```python
from build123d import *

# Parameters (mm, degrees)
SKETCH1_W           = 95.192719723
SKETCH1_H           = 77.236030742
BOSS_EXTRUDE1_DEPTH = 5
SKETCH2_W           = 20.458340989
SKETCH2_H           = 77.236030742
BOSS_EXTRUDE2_DEPTH = 2
SKETCH3_W           = 97.192719723
SKETCH3_H           = 20.458340989
BOSS_EXTRUDE3_DEPTH = 2
SKETCH4_W           = 97.192719723
SKETCH4_H           = 20.458340989
BOSS_EXTRUDE4_DEPTH = 2
LPATTERN1_COUNT     = 6
LPATTERN1_PITCH     = 19.038543945
CUT_EXTRUDE1_REACH  = 115.159
SKETCH7_W           = 11.458340989
SKETCH7_H           = 3.5


with BuildPart() as part:
    # Sketch1 → Boss-Extrude1 (new body)
    with BuildSketch(Plane.XY):
        with Locations((47.596359862, -38.618015371)):
            Rectangle(SKETCH1_W, SKETCH1_H)
    extrude(amount=BOSS_EXTRUDE1_DEPTH)

    # Sketch2 → Boss-Extrude2 (add)
    with BuildSketch(Plane.ZY):
        with Locations((10.229170494, -38.618015371)):
            Rectangle(SKETCH2_W, SKETCH2_H)
    boss_extrude2 = extrude(amount=BOSS_EXTRUDE2_DEPTH)

    # Sketch3 → Boss-Extrude3 (add)
    with BuildSketch(Plane(origin=(0, 0, 0), x_dir=(1, 0, 0), z_dir=(0, 1, 0))):
        with Locations((46.596359862, -10.229170494)):
            Rectangle(SKETCH3_W, SKETCH3_H)
    extrude(amount=BOSS_EXTRUDE3_DEPTH)

    # Sketch4 → Boss-Extrude4 (add)
    with BuildSketch(Plane.XZ.offset(77.236030742)):
        with Locations((46.596359862, 10.229170494)):
            Rectangle(SKETCH4_W, SKETCH4_H)
    extrude(amount=BOSS_EXTRUDE4_DEPTH)

    # LPattern1: Boss-Extrude2 ×6
    with Locations(*[(i * LPATTERN1_PITCH, 0, 0) for i in range(1, LPATTERN1_COUNT)]):
        add(boss_extrude2)

    # Cut-Extrude1: up to this face of the body (flat: up to its plane)
    cut_extrude1_end = Plane(part.part.faces().sort_by_distance((76.154175778, -38.618015371, 12.729170494))[0])
    # Sketch7 → Cut-Extrude1 (cut, up to the picked face)
    with BuildSketch(Plane.ZY.offset(-17.038543945), mode=Mode.PRIVATE) as cut_extrude1_sk1:
        with Locations((12.729170494, -1.75)):
            Rectangle(SKETCH7_W, SKETCH7_H)
    cut_extrude1_tool1 = split(extrude(cut_extrude1_sk1.sketch, amount=-CUT_EXTRUDE1_REACH, mode=Mode.PRIVATE), bisect_by=cut_extrude1_end, keep=Keep.BOTH, mode=Mode.PRIVATE)
    # Sketch7 → Cut-Extrude1 (cut, up to the picked face)
    with BuildSketch(Plane.ZY.offset(-17.038543945), mode=Mode.PRIVATE) as cut_extrude1_sk2:
        with Locations((12.729170494, -75.486030742)):
            Rectangle(SKETCH7_W, SKETCH7_H)
    cut_extrude1_tool2 = split(extrude(cut_extrude1_sk2.sketch, amount=-CUT_EXTRUDE1_REACH, mode=Mode.PRIVATE), bisect_by=cut_extrude1_end, keep=Keep.BOTH, mode=Mode.PRIVATE)
    add(cut_extrude1_tool1.solids().sort_by(Axis((17.038544, -1.75, 12.72917), (1, 0, 0)))[0], mode=Mode.SUBTRACT)
    add(cut_extrude1_tool2.solids().sort_by(Axis((17.038544, -75.486031, 12.72917), (1, 0, 0)))[0], mode=Mode.SUBTRACT)


solid = part.part
```
Geometry check sheet. Reference: the model listing, model coordinates, mm. A direction names the side the tool comes from. Round coordinates to 2 decimals unless told otherwise and drop trailing zeros. Order: outer loops, then holes, each group sorted by start corner. A loop starts at its lowest first (then second) coordinate and runs counter-clockwise, first axis right, second up. Notation, with made-up numbers: (21, -5.5) - (70, -5.5) arc R24 ccw to (70, 6.5) - close; hole circle Ø9 at (-11.75, 27.25). An arc over 180 degrees is marked (long way). Use a Markdown table: item, result. Add a question column.
1) Thickness scan on line 1 along X through (y, z) = (-73, 16.75); line 2 along Y through (x, z) = (56.5, 17.75); line 3 along Y through (x, z) = (87, 10.5). Record the ranges inside material, lowest first.
2) Mould release check, pull along Z, two halves, no side actions. Record for faces 1 (the flat face through (46, 2, 10)), 2 (the flat face through (18, -76, 18.458)), 3 (the flat face through (8, -38, 5)): released by +Z, released by -Z, zero draft, split by the parting line, or undercut.
3) Set-up check for faces 4 (the flat face through (75, -3.5, 13)), 5 (the flat face through (19.039, -38, 13)): record each of +Z, -Z, +X, -X, +Y, -Y from which the full face is reachable in a straight line by a thin tool's end or side.
4) Section check C-C (x = 61.5). Record the cut outline in (y, z), then the cut area to 3 significant figures.
5) Section check B-B (y = -54). Record the cut outline in (x, z), then the cut area to 3 significant figures.
6) Section check A-A (z = 15.5). Record the cut outline in (x, y).
7) Gauge pin test, flat ends, axial feed: P1, Ø6, axis at x = 13.5, y = -68.5, coming from the +Z side; P2, Ø18.5, axis at x = 46.5, y = -48.5, coming from the +Z side. Record the tip position at first contact, or that the pin passes through.
Established:
| question | item | result |
|---|---|---|
| 1 | line 1 | -2 to 0, 17.04 to 19.04, 36.08 to 38.08, 55.12 to 57.12, 74.15 to 76.15, 93.19 to 95.19 |
| 1 | line 2 | -79.24 to -77.24, -73.74 to -3.5, 0 to 2 |
| 1 | line 3 | -79.24 to -77.24, 0 to 2 |
| 2 | face 1 | zero draft |
| 2 | face 2 | undercut |
| 2 | face 3 | released by +Z |
| 3 | face 4 | none |
| 3 | face 5 | +Z |
| 4 | outline | (-79.24, 0) - (2, 0) - (2, 20.46) - (0, 20.46) - (0, 5) - (-77.24, 5) - (-77.24, 20.46) - (-79.24, 20.46) - close |
| 4 | area | 468 mm2 |
| 5 | outline | (-2, 0) - (95.19, 0) - (95.19, 20.46) - (93.19, 20.46) - (93.19, 5) - (76.15, 5) - (76.15, 20.46) - (74.15, 20.46) - (74.15, 5) - (57.12, 5) - (57.12, 20.46) - (55.12, 20.46) - (55.12, 5) - (38.08, 5) - (38.08, 20.46) - (36.08, 20.46) - (36.08, 5) - (19.04, 5) - (19.04, 20.46) - (17.04, 20.46) - (17.04, 5) - (0, 5) - (0, 20.46) - (-2, 20.46) - close |
| 5 | area | 671 mm2 |
| 6 | outline | (-2, -79.24) - (95.19, -79.24) - (95.19, 2) - (-2, 2) - close; (17.04, -73.74) - (19.04, -73.74) - (19.04, -3.5) - (17.04, -3.5) - close; (36.08, -73.74) - (38.08, -73.74) - (38.08, -3.5) - (36.08, -3.5) - close; (55.12, -73.74) - (57.12, -73.74) - (57.12, -3.5) - (55.12, -3.5) - close; (74.15, -73.74) - (76.15, -73.74) - (76.15, -3.5) - (74.15, -3.5) - close; hole (0, -77.24) - (93.19, -77.24) - (93.19, 0) - (0, 0) - close |
| 7 | P1 | z = 5 |
| 7 | P2 | z = 20.46 |
